```python
from build123d import *

# Parameters (mm, degrees)
F1_DEPTH  = 103.759
F2_W      = 5.207
F2_H      = 2.8575
F2_H_2    = 16.2052
F2_H_3    = 2.9408035447
F3_DEPTH  = 2.9972
F4_R      = 2.54
F5_DEPTH  = 12.7
F6_R      = 4.6
F7_DEPTH  = 25.4
F8_R      = 4.6
F9_DEPTH  = 25.4
F10_R     = 4.6
F11_DEPTH = 25.4
F13_DEPTH = 127
F14_R     = 4.699
F15_DEPTH = 2
F16_R     = 4.699
F17_DEPTH = 2
F18_DEPTH = 25.4
F19_R     = 4.699
F20_DEPTH = 2
F21_DEPTH = 25.4
F22_SIZE  = 0.8


with BuildPart() as f1:
    # F0 (on Right) → F1 (new body)
    with BuildSketch(Plane.YZ):
        Polygon((0, 1.524), (0, 0), (16.2052, 0), (16.2052, 1.524), (19.0627, 4.3815), (16.2052, 7.239), (0, 7.239), (-2.8575, 4.3815), align=None)
    extrude(amount=F1_DEPTH)

    # F2 (on face) → F3 (cut)
    with BuildSketch(Plane.XY.offset(7.239)):
        with Locations((7.3025, -1.42875)):
            Rectangle(F2_W, F2_H)
        Polygon((4.699, 16.2052), (4.699, 8.1026), (4.699, 0), (9.906, 0), (9.906, 16.2052), align=None)
        with Locations((7.3025, 17.63395)):
            Rectangle(F2_W, F2_H)
        with Locations((17.2085, 17.63395)):
            Rectangle(F2_W, F2_H)
        with Locations((17.2085, 8.1026)):
            Rectangle(F2_W, F2_H_2)
        with Locations((17.2085, -1.42875)):
            Rectangle(F2_W, F2_H)
        with Locations((27.1145, 17.63395)):
            Rectangle(F2_W, F2_H)
        with Locations((27.1145, 8.1026)):
            Rectangle(F2_W, F2_H_2)
        with Locations((27.1145, -1.42875)):
            Rectangle(F2_W, F2_H)
        with Locations((37.0205, 17.63395)):
            Rectangle(F2_W, F2_H)
        with Locations((37.0205, 8.1026)):
            Rectangle(F2_W, F2_H_2)
        with Locations((37.0205, -1.42875)):
            Rectangle(F2_W, F2_H)
        with Locations((46.9265, 17.63395)):
            Rectangle(F2_W, F2_H)
        with Locations((46.9265, 8.1026)):
            Rectangle(F2_W, F2_H_2)
        with Locations((46.9265, -1.42875)):
            Rectangle(F2_W, F2_H)
        with Locations((56.8325, 17.63395)):
            Rectangle(F2_W, F2_H)
        with Locations((56.8325, 8.1026)):
            Rectangle(F2_W, F2_H_2)
        with Locations((56.8325, -1.42875)):
            Rectangle(F2_W, F2_H)
        with Locations((66.7385, 17.63395)):
            Rectangle(F2_W, F2_H)
        with Locations((66.7385, 8.1026)):
            Rectangle(F2_W, F2_H_2)
        with Locations((66.7385, -1.42875)):
            Rectangle(F2_W, F2_H)
        with Locations((76.6445, 17.63395)):
            Rectangle(F2_W, F2_H)
        with Locations((76.6445, 8.1026)):
            Rectangle(F2_W, F2_H_2)
        with Locations((76.6445, -1.42875)):
            Rectangle(F2_W, F2_H)
        with Locations((86.5505, -1.42875)):
            Rectangle(F2_W, F2_H)
        with Locations((86.5505, 8.1026)):
            Rectangle(F2_W, F2_H_2)
        with Locations((86.5505, 17.63395)):
            Rectangle(F2_W, F2_H)
        with Locations((96.4565, 17.6756017723)):
            Rectangle(F2_W, F2_H_3)
        with Locations((96.4565, 8.1026)):
            Rectangle(F2_W, F2_H_2)
        with Locations((96.4565, -1.4704017723)):
            Rectangle(F2_W, F2_H_3)
    extrude(amount=-F3_DEPTH, mode=Mode.SUBTRACT)

    # F4 (on face) → F5 (cut, symmetric)
    with BuildSketch(Plane(origin=(0, 0, 0), x_dir=(1, 0, 0), z_dir=(0, 0, -1))):
        with Locations((87.503, -8.3177030837)):
            Circle(F4_R)
        with Locations((16.383, -8.1026)):
            Circle(F4_R)
        with Locations((51.943, -8.3177030837)):
            Circle(F4_R)
    extrude(amount=F5_DEPTH, both=True, mode=Mode.SUBTRACT)

    # F6 (on face) → F7 (cut)
    with BuildSketch(Plane.XY.offset(4.2418)):
        with Locations((16.383, 8.1026)):
            Circle(F6_R)
    extrude(amount=F7_DEPTH, mode=Mode.SUBTRACT)

    # F8 (on face) → F9 (cut)
    with BuildSketch(Plane.XY.offset(4.2418)):
        with Locations((87.503, 8.3177030837)):
            Circle(F8_R)
    extrude(amount=F9_DEPTH, mode=Mode.SUBTRACT)

    # F10 (on face) → F11 (cut)
    with BuildSketch(Plane.XY.offset(4.2418)):
        with Locations((51.943, 8.3177030837)):
            Circle(F10_R)
    extrude(amount=F11_DEPTH, mode=Mode.SUBTRACT)

    # F12 (on face) → F13 (cut)
    with BuildSketch(Plane.YZ.offset(103.759)):
        Polygon((0.6026, 0.9214), (-2.8575, 4.3815), (-2.8575, 0), (0.6026, 0), align=None)
        Polygon((19.0627, 0), (19.0627, 4.3815), (15.6026, 0.9214), (15.6026, 0), align=None)
    extrude(amount=-F13_DEPTH, mode=Mode.SUBTRACT)

    # F14 (on face) → F15 (cut)
    with BuildSketch(Plane.XY.offset(4.2418)):
        with Locations((16.383, 8.1026)):
            Circle(F14_R)
    extrude(amount=-F15_DEPTH, mode=Mode.SUBTRACT)

    # F16 (on face) → F17 (cut)
    with BuildSketch(Plane.XY.offset(4.2418)):
        with Locations((51.943, 8.3177030837)):
            Circle(F16_R)
    extrude(amount=-F17_DEPTH, mode=Mode.SUBTRACT)

    # F16 (on face) → F18 (cut)
    with BuildSketch(Plane.XY.offset(4.2418)):
        with Locations((51.943, 8.3177030837)):
            Circle(F16_R)
    extrude(amount=F18_DEPTH, mode=Mode.SUBTRACT)

    # F19 (on face) → F20 (cut)
    with BuildSketch(Plane.XY.offset(4.2418)):
        with Locations((87.503, 8.3177030837)):
            Circle(F19_R)
    extrude(amount=-F20_DEPTH, mode=Mode.SUBTRACT)

    # F19 (on face) → F21 (cut)
    with BuildSketch(Plane.XY.offset(4.2418)):
        with Locations((87.503, 8.3177030837)):
            Circle(F19_R)
    extrude(amount=F21_DEPTH, mode=Mode.SUBTRACT)

    # F22
    f22_edges = [f1.edges().sort_by_distance(p)[0] for p in [
        (84.963, 8.317703, 2.2418),
        (49.403, 8.317703, 2.2418),
        (13.843, 8.1026, 2.2418),
    ]]
    chamfer(f22_edges, length=F22_SIZE)


solid = f1.part
```
For this review, take the finished solid that the model builds, in its own axes (mm). A direction names the side the tool comes from. Coordinates: 2 decimals unless noted, no trailing zeros.
(1) For pin 1 Ø8 at (x, y) = (16.38, 8.1) entering from +Z; pin 2 Ø4 at (x, y) = (76.5, 13) entering from +Z; pin 3 Ø5.5 at (x, y) = (16.38, 8.1) entering from +Z; pin 4 Ø0.9 at (y, z) = (5.5, 5) entering from -X, all flat-tipped, find the tip position at first contact; note any pin that passes through.
(2) Wall thickness on probe 1 along Z at (x, y) = (47, 6.75); probe 2 along X at (y, z) = (9.5, 2.5); probe 3 along X at (y, z) = (7.25, 0.5): over which ranges is each line inside the solid? List them lowest first.
(3) The part is to be moulded in two halves that separate along X. For faces 4 (the face through (18.729, 9.075, 0.711)), 5 (the face through (32.035, 17.654, 5.79)), say which applies: +X half, -X half, draft (parallel to the pull), parting line (faces both ways), or undercut.
(4) Tool access review of faces 1 (the face through (11.69, 8.31, 3.26)), 2 (the face through (52, 14, 7.239)), 3 (the face through (89.154, 15, 6)): name each direction out of +Z, -Z, +X, -X, +Y, -Y from which nothing blocks a thin tool from reaching the whole face with its end or side.
(5) Add section A-A on y = 6.75. Count the separate pieces of the cut face and the enclosed holes in it, then the cut area to 3 significant figures.
Answer sheet:
1. pin 1: stops at z = 2.24
1. pin 2: stops at z = 4.24
1. pin 3: stops at z = 1.66
1. pin 4: stops at x = 0
2. probe 1: z = 0 to 4.24
2. probe 2: x = 0 to 11.9, 20.87 to 47.4, 56.49 to 82.96, 92.05 to 103.76
2. probe 3: x = 0 to 13.99, 18.78 to 49.64, 54.25 to 85.2, 89.81 to 103.76
3. face 4: undercut
3. face 5: draft
4. face 1: none
4. face 2: +Z, +X, -X, +Y, -Y
4. face 3: +Z, +Y, -Y
5. separate pieces: 4
5. enclosed holes: 0
5. area: 476 mm2
